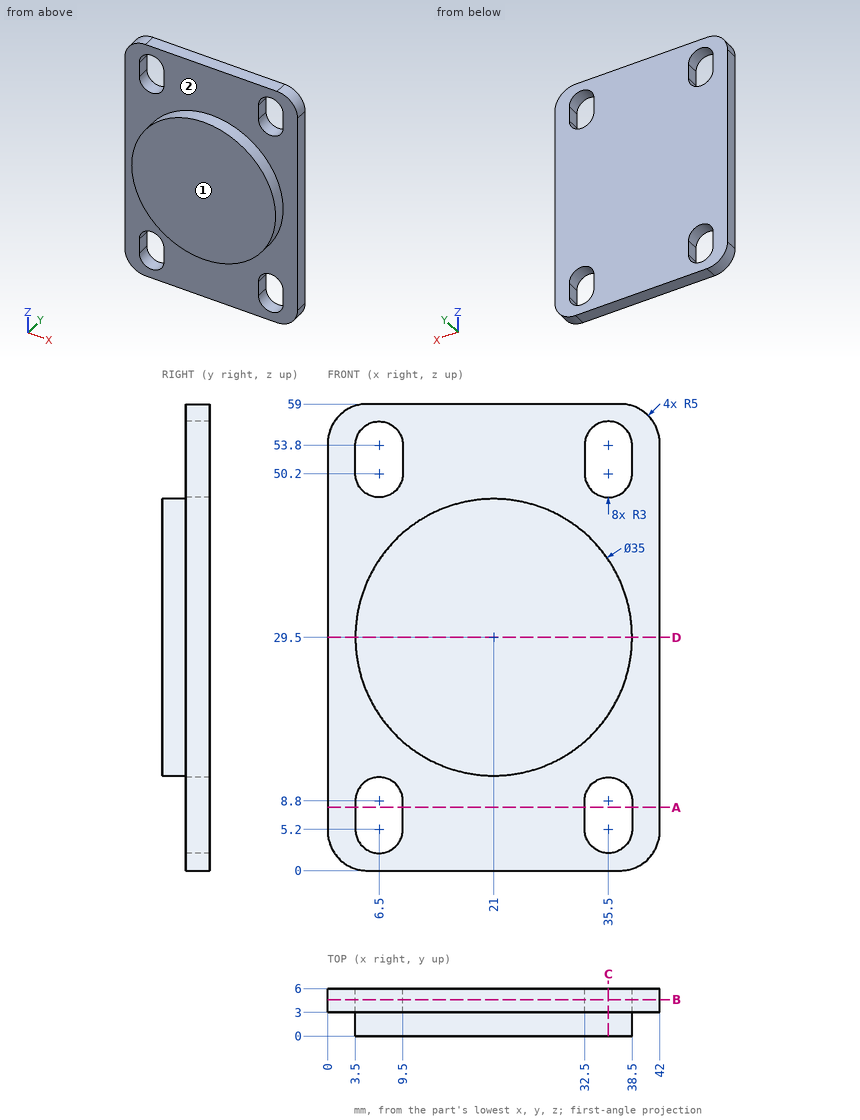
Can you work these out from the drawing? Everything is in mm from the part's minimum corner. A direction names the side the tool comes from. Give positions to 0.01 mm unless a question says otherwise; leave off trailing zeros. Order: outer loops, then holes, each group sorted by start corner. A loop starts at its lowest first (then second) coordinate and runs counter-clockwise, first axis right, second up. Notation, with made-up numbers: M 20.5,56 L 34.5,56 A25 cw 34.5,68 Z; hole C 15.5,31.25 d7. An arc over 180 degrees is marked long. One line per item, written item: value.
Item 1: If we section it at D-D on z = 29.5: Write out the boundary of the cut face in (x, y).
Verdict:
outline: M 0,3 L 3.5,3 L 3.5,0 L 38.5,0 L 38.5,3 L 42,3 L 42,6 L 0,6 Z
Item 2: For pin 1 (1.5 mm diameter, centred on x = 12, z = 10.5, fed in from -Y); pin 2 (2.5 mm diameter, centred on y = 4, z = 52.5, fed in from -X), each with a flat end and sliding along its axis, tell me the tip position at first contact or that it passes through.
Verdict:
pin 1: y = 3
pin 2: x = 0
Item 3: If we section it at C-C on x = 35.5: Write out the boundary of the cut face in (y, z).
Verdict:
outline: M 0,19.7 L 3,19.7 L 3,11.8 L 6,11.8 L 6,47.2 L 3,47.2 L 3,39.3 L 0,39.3 Z; M 3,0 L 6,0 L 6,2.2 L 3,2.2 Z; M 3,56.8 L 6,56.8 L 6,59 L 3,59 Z
Item 4: If we section it at A-A on z = 8: Write out the boundary of the cut face in (x, y), and give its area (3 significant figures).
Verdict:
outline: M 0,3 L 3.5,3 L 3.5,6 L 0,6 Z; M 9.5,3 L 32.5,3 L 32.5,6 L 9.5,6 Z; M 38.5,3 L 42,3 L 42,6 L 38.5,6 Z
area: 90.0 mm2
Item 5: Please list where these lines run through material, in increasing order: line 1 (X direction, y = 3.4, z = 8.5); line 2 (X direction, y = 3.4, z = 10); line 3 (Y direction, x = 2, z = 45.5).
Verdict:
line 1: 0 to 3.5, 9.5 to 32.5, 38.5 to 42
line 2: 0 to 3.75, 9.25 to 32.75, 38.25 to 42
line 3: 3 to 6
Item 6: If we section it at B-B on y = 4.6: Write out the boundary of the cut face in (x, z).
Verdict:
outline: M 0,5 A5 ccw 5,0 L 37,0 A5 ccw 42,5 L 42,54 A5 ccw 37,59 L 5,59 A5 ccw 0,54 Z; hole M 3.5,5.2 A3 ccw 9.5,5.2 L 9.5,8.8 A3 ccw 3.5,8.8 Z; hole M 3.5,50.2 A3 ccw 9.5,50.2 L 9.5,53.8 A3 ccw 3.5,53.8 Z; hole M 32.5,5.2 A3 ccw 38.5,5.2 L 38.5,8.8 A3 ccw 32.5,8.8 Z; hole M 32.5,50.2 A3 ccw 38.5,50.2 L 38.5,53.8 A3 ccw 32.5,53.8 Z
Item 7: For the marked faces 1 and 2, which set-ups out of +Z, -Z, +X, -X, +Y, -Y let a thin tool reach every point of the face, with its end or its side?
Verdict:
face 1: +Z, -Z, +X, -X, -Y
face 2: -Y
